Design review of the part built by this model. Coordinates are the model's own, in mm. Give positions to 0.01 mm unless a question says otherwise; leave off trailing zeros. Loops run counter-clockwise (first coordinate to the right, second up) from the corner with the lowest first, then second, coordinate; pieces in that order, holes last. Notation, with made-up numbers: (74.25, 56.25) - (115.25, 56.25) arc R22 cw to (115.25, 76.25) - close; hole circle Ø10 at (-11, -36). An arc over 180 degrees is marked (long way). Put each result on its own line as item: value. Start each with the question number.
```python
from build123d import *

# Parameters (mm, degrees)
F0_W         = 62.5
F0_H         = 25
F0_W_2       = 25
F0_H_2       = 62.5
F1_DEPTH     = 2
F2_T1_DEPTH  = 69.5710678119
F2_T3_DEPTH  = 69.5710678119
F2_T5_DEPTH  = 39.1421356237
F2_T7_DEPTH  = 69.5710678119
F2_T9_DEPTH  = 39.1421356237
F2_T11_DEPTH = 69.5710678119
F2_T17_DEPTH = 69.5710678119
F2_T21_DEPTH = 69.5710678119
F2_T28_DEPTH = 69.5710678119
F2_T32_DEPTH = 69.5710678119
F2_T39_DEPTH = 69.5710678119
F2_T43_DEPTH = 69.5710678119
F2_T50_DEPTH = 69.5710678119
F2_T54_DEPTH = 69.5710678119


# Not quite as in the source:
# - a fillet or chamfer that OpenCascade refuses, or shapes differently, is made with other operations: its cross-section is extruded or revolved along the edge and cut away or added
# - a feature names something its author has since deleted; it is built from what else it names


with BuildPart() as f1:
    # F0 (on Top) → F1 (new body)
    with BuildSketch(Plane.XY):
        with Locations((-43.75, 0)):
            Rectangle(F0_W, F0_H)
        Rectangle(F0_W_2, F0_H)
        with Locations((0, -43.75)):
            Rectangle(F0_W_2, F0_H_2)
        with Locations((0, 43.75)):
            Rectangle(F0_W_2, F0_H_2)
        with Locations((43.75, 0)):
            Rectangle(F0_W, F0_H)
    extrude(amount=F1_DEPTH)

    # F2: fillet of radius 3 on 12 edges, made by hand

    # F2_s2 → F2_t1 (cut)
    with BuildSketch(Plane.YZ.offset(-82.0710678119)):
        with BuildLine():
            ThreePointArc((-12.5, 2), (-11.4036236828, 0.5505102572), (-9.6715728753, 0))
            Line((-9.6715728753, 0), (-12.5, 0))
            Line((-12.5, 0), (-12.5, 2))
        make_face()
        with BuildLine():
            ThreePointArc((12.5, 2), (11.4036236828, 0.5505102572), (9.6715728753, 0))
            Line((9.6715728753, 0), (12.5, 0))
            Line((12.5, 0), (12.5, 2))
        make_face()
    extrude(amount=F2_T1_DEPTH, mode=Mode.SUBTRACT)

    # F2_s4 → F2_t3 (cut)
    with BuildSketch(Plane.XZ.offset(12.5)):
        with BuildLine():
            ThreePointArc((-12.5, 2), (-11.4036236828, 0.5505102572), (-9.6715728753, 0))
            Line((-9.6715728753, 0), (-12.5, 0))
            Line((-12.5, 0), (-12.5, 2))
        make_face()
        with BuildLine():
            ThreePointArc((12.5, 2), (11.4036236828, 0.5505102572), (9.6715728753, 0))
            Line((9.6715728753, 0), (12.5, 0))
            Line((12.5, 0), (12.5, 2))
        make_face()
    extrude(amount=F2_T3_DEPTH, mode=Mode.SUBTRACT)

    # F2_s6 → F2_t5 (cut)
    with BuildSketch(Plane.YZ.offset(-19.5710678119)):
        with BuildLine():
            ThreePointArc((-75, 2), (-73.9036236828, 0.5505102572), (-72.1715728753, 0))
            Line((-72.1715728753, 0), (-75, 0))
            Line((-75, 0), (-75, 2))
        make_face()
        with BuildLine():
            ThreePointArc((75, 2), (73.9036236828, 0.5505102572), (72.1715728753, 0))
            Line((72.1715728753, 0), (75, 0))
            Line((75, 0), (75, 2))
        make_face()
    extrude(amount=F2_T5_DEPTH, mode=Mode.SUBTRACT)

    # F2_s8 → F2_t7 (cut)
    with BuildSketch(Plane.YZ.offset(12.5)):
        with BuildLine():
            ThreePointArc((-12.5, 2), (-11.4036236828, 0.5505102572), (-9.6715728753, 0))
            Line((-9.6715728753, 0), (-12.5, 0))
            Line((-12.5, 0), (-12.5, 2))
        make_face()
        with BuildLine():
            ThreePointArc((12.5, 2), (11.4036236828, 0.5505102572), (9.6715728753, 0))
            Line((9.6715728753, 0), (12.5, 0))
            Line((12.5, 0), (12.5, 2))
        make_face()
    extrude(amount=F2_T7_DEPTH, mode=Mode.SUBTRACT)

    # F2_s10 → F2_t9 (cut)
    with BuildSketch(Plane.XZ.offset(-19.5710678119)):
        with BuildLine():
            ThreePointArc((75, 2), (73.9036236828, 0.5505102572), (72.1715728753, 0))
            Line((72.1715728753, 0), (75, 0))
            Line((75, 0), (75, 2))
        make_face()
        with BuildLine():
            ThreePointArc((-75, 2), (-73.9036236828, 0.5505102572), (-72.1715728753, 0))
            Line((-72.1715728753, 0), (-75, 0))
            Line((-75, 0), (-75, 2))
        make_face()
    extrude(amount=F2_T9_DEPTH, mode=Mode.SUBTRACT)

    # F2_s12 → F2_t11 (cut)
    with BuildSketch(Plane.XZ.offset(-82.0710678119)):
        with BuildLine():
            ThreePointArc((12.5, 2), (11.4036236828, 0.5505102572), (9.6715728753, 0))
            Line((9.6715728753, 0), (12.5, 0))
            Line((12.5, 0), (12.5, 2))
        make_face()
        with BuildLine():
            ThreePointArc((-12.5, 2), (-11.4036236828, 0.5505102572), (-9.6715728753, 0))
            Line((-9.6715728753, 0), (-12.5, 0))
            Line((-12.5, 0), (-12.5, 2))
        make_face()
    extrude(amount=F2_T11_DEPTH, mode=Mode.SUBTRACT)


with BuildPart() as f2_tool15:
    # F2_s16 → F2_t17 (new body)
    with BuildSketch(Plane.YZ.offset(-75)):
        with BuildLine():
            ThreePointArc((-12.5, 2), (-11.4036236828, 0.5505102572), (-9.6715728753, 0))
            Line((-9.6715728753, 0), (-12.5, 0))
            Line((-12.5, 0), (-12.5, 2))
        make_face()
    extrude(amount=F2_T17_DEPTH)

    split(bisect_by=Plane.YZ.offset(-12.5), keep=Keep.TOP)


with BuildPart() as f2_tool19:
    # F2_s20 → F2_t21 (new body)
    with BuildSketch(Plane.XZ.offset(5.4289321881)):
        with BuildLine():
            ThreePointArc((-12.5, 2), (-11.4036236828, 0.5505102572), (-9.6715728753, 0))
            Line((-9.6715728753, 0), (-12.5, 0))
            Line((-12.5, 0), (-12.5, 2))
        make_face()
    extrude(amount=F2_T21_DEPTH)

    split(bisect_by=Plane.XZ.offset(12.5), keep=Keep.BOTTOM)


with BuildPart() as f2_tool15_1:
    add(f2_tool15.part)

    # F2_t23: intersect F2_tool19
    add(f2_tool19.part, mode=Mode.INTERSECT)


with BuildPart() as f1_1:
    add(f1.part)

    # F2_t13: cut F2_tool15
    add(f2_tool15_1.part, mode=Mode.SUBTRACT)


with BuildPart() as f2_tool26:
    # F2_s27 → F2_t28 (new body)
    with BuildSketch(Plane.XZ.offset(75)):
        with BuildLine():
            ThreePointArc((12.5, 2), (11.4036236828, 0.5505102572), (9.6715728753, 0))
            Line((9.6715728753, 0), (12.5, 0))
            Line((12.5, 0), (12.5, 2))
        make_face()
    extrude(amount=-F2_T28_DEPTH)

    split(bisect_by=Plane.XZ.offset(12.5), keep=Keep.BOTTOM)


with BuildPart() as f2_tool30:
    # F2_s31 → F2_t32 (new body)
    with BuildSketch(Plane.YZ.offset(5.4289321881)):
        with BuildLine():
            ThreePointArc((-12.5, 2), (-11.4036236828, 0.5505102572), (-9.6715728753, 0))
            Line((-9.6715728753, 0), (-12.5, 0))
            Line((-12.5, 0), (-12.5, 2))
        make_face()
    extrude(amount=F2_T32_DEPTH)

    split(bisect_by=Plane.YZ.offset(12.5), keep=Keep.BOTTOM)


with BuildPart() as f2_tool26_1:
    add(f2_tool26.part)

    # F2_t34: intersect F2_tool30
    add(f2_tool30.part, mode=Mode.INTERSECT)


with BuildPart() as f1_2:
    add(f1_1.part)

    # F2_t24: cut F2_tool26
    add(f2_tool26_1.part, mode=Mode.SUBTRACT)


with BuildPart() as f2_tool37:
    # F2_s38 → F2_t39 (new body)
    with BuildSketch(Plane.YZ.offset(75)):
        with BuildLine():
            ThreePointArc((12.5, 2), (11.4036236828, 0.5505102572), (9.6715728753, 0))
            Line((9.6715728753, 0), (12.5, 0))
            Line((12.5, 0), (12.5, 2))
        make_face()
    extrude(amount=-F2_T39_DEPTH)

    split(bisect_by=Plane.YZ.offset(12.5), keep=Keep.BOTTOM)


with BuildPart() as f2_tool41:
    # F2_s42 → F2_t43 (new body)
    with BuildSketch(Plane.XZ.offset(-5.4289321881)):
        with BuildLine():
            ThreePointArc((12.5, 2), (11.4036236828, 0.5505102572), (9.6715728753, 0))
            Line((9.6715728753, 0), (12.5, 0))
            Line((12.5, 0), (12.5, 2))
        make_face()
    extrude(amount=-F2_T43_DEPTH)

    split(bisect_by=Plane.XZ.offset(-12.5), keep=Keep.TOP)


with BuildPart() as f2_tool37_1:
    add(f2_tool37.part)

    # F2_t45: intersect F2_tool41
    add(f2_tool41.part, mode=Mode.INTERSECT)


with BuildPart() as f1_3:
    add(f1_2.part)

    # F2_t35: cut F2_tool37
    add(f2_tool37_1.part, mode=Mode.SUBTRACT)


with BuildPart() as f2_tool48:
    # F2_s49 → F2_t50 (new body)
    with BuildSketch(Plane.XZ.offset(-75)):
        with BuildLine():
            ThreePointArc((-12.5, 2), (-11.4036236828, 0.5505102572), (-9.6715728753, 0))
            Line((-9.6715728753, 0), (-12.5, 0))
            Line((-12.5, 0), (-12.5, 2))
        make_face()
    extrude(amount=F2_T50_DEPTH)

    split(bisect_by=Plane.XZ.offset(-12.5), keep=Keep.TOP)


with BuildPart() as f2_tool52:
    # F2_s53 → F2_t54 (new body)
    with BuildSketch(Plane.YZ.offset(-5.4289321881)):
        with BuildLine():
            ThreePointArc((12.5, 2), (11.4036236828, 0.5505102572), (9.6715728753, 0))
            Line((9.6715728753, 0), (12.5, 0))
            Line((12.5, 0), (12.5, 2))
        make_face()
    extrude(amount=-F2_T54_DEPTH)

    split(bisect_by=Plane.YZ.offset(-12.5), keep=Keep.TOP)


with BuildPart() as f2_tool48_1:
    add(f2_tool48.part)

    # F2_t56: intersect F2_tool52
    add(f2_tool52.part, mode=Mode.INTERSECT)


with BuildPart() as f1_4:
    add(f1_3.part)

    # F2_t46: cut F2_tool48
    add(f2_tool48_1.part, mode=Mode.SUBTRACT)


solid = f1_4.part
```
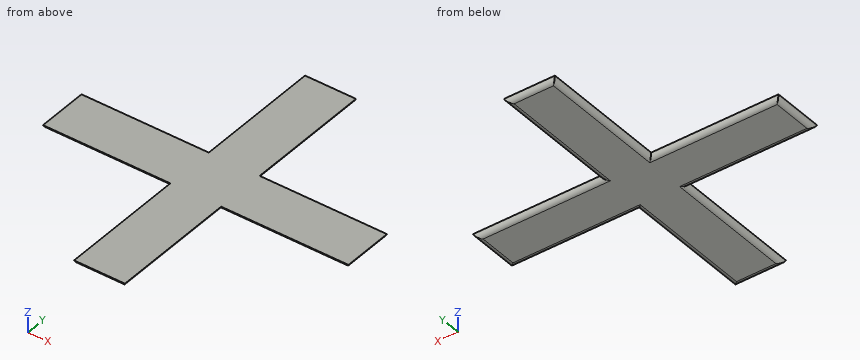
Item 1: For P1, Ø5, axis at x = -27, y = 16, coming from the +Z side, flat-tipped, find the tip position at first contact; note if it passes through.
Item 2: For L1, parallel to Y at x = -6, z = 1.95; L2, parallel to X at y = -41.5, z = 0.8; L3, parallel to Y at x = 64, z = 0.3, list the stretches that pass through material, from the lowest coordinate up. Write a range as from..to.
Item 3: Consider section A-A (z = 1.05). State the section outline as (x, y) points, plus the area to 3 significant figures.
Item 4: Consider section B-B (x = -34). State the section outline as (y, z) points.
Geometry says:
1. P1: passes through
2. L1: y = -74.98..74.98
2. L2: x = -11.71..11.71
2. L3: y = -10.98..10.98
3. outline: (-74.45, -11.95) - (-11.95, -11.95) - (-11.95, -74.45) - (11.95, -74.45) - (11.95, -11.95) - (74.45, -11.95) - (74.45, 11.95) - (11.95, 11.95) - (11.95, 74.45) - (-11.95, 74.45) - (-11.95, 11.95) - (-74.45, 11.95) - close
3. area: 6,550 mm2
4. outline: (-12.5, 2) arc R3 ccw to (-9.67, 0) - (9.67, 0) arc R3 ccw to (12.5, 2) - close
